Can you work these out from the model? Positions are in its coordinate system, mm. Face numbers are marked on the shaded views. A direction names the side the tool comes from. Give positions to 0.01 mm unless a question says otherwise; leave off trailing zeros. Order: outer loops, then holes, each group sorted by start corner. A loop starts at its lowest first (then second) coordinate and runs counter-clockwise, first axis right, second up. Notation, with made-up numbers: (-19, 49.5) -> (-9, 49.5) arc R31 cw to (-9, 73.5) -> close; hole circle Ø11 at (71, -1.5). An arc over 180 degrees is marked (long way). Answer as CSV lines item,"result".
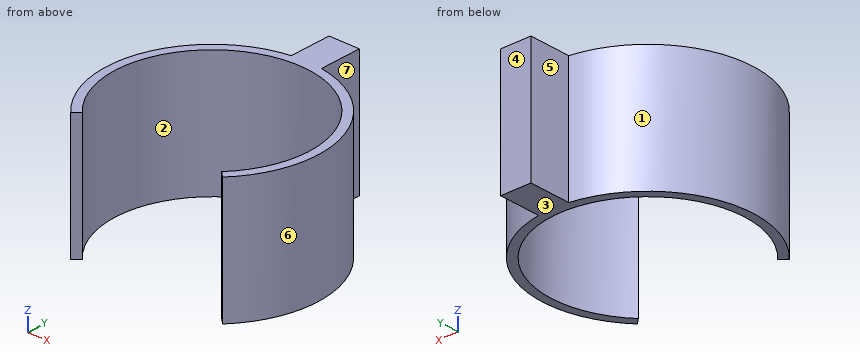
```python
from build123d import *

# Parameters (mm, degrees)
SKETCH1_R           = 4.25
SKETCH1_R_2         = 3.9
BOSS_EXTRUDE1_DEPTH = 5
CUT_EXTRUDE1_DEPTH  = 5
SKETCH3_W           = 1.224263259
SKETCH3_H           = 5
BOSS_EXTRUDE2_DEPTH = 2


with BuildPart() as part:
    # Sketch1 → Boss-Extrude1 (new body)
    with BuildSketch(Plane.XY):
        Circle(SKETCH1_R)
        Circle(SKETCH1_R_2, mode=Mode.SUBTRACT)
    extrude(amount=BOSS_EXTRUDE1_DEPTH)

    # Sketch2 → Cut-Extrude1 (cut)
    with BuildSketch(Plane.XY.offset(5)):
        with BuildLine():
            Line((-3.074069072, -2.934723044), (-2.820910442, -2.69303997))
            ThreePointArc((-2.820910442, -2.69303997), (0, -3.9), (2.820910442, -2.69303997))
            Line((2.820910442, -2.69303997), (3.074069072, -2.934723044))
            ThreePointArc((3.074069072, -2.934723044), (0, -4.25), (-3.074069072, -2.934723044))
        make_face()
    extrude(amount=-CUT_EXTRUDE1_DEPTH, mode=Mode.SUBTRACT)

    # Sketch3 → Boss-Extrude2 (add)
    with BuildSketch(Plane(origin=(0, 3.9, 0), x_dir=(1, 0, 0), z_dir=(0, 1, 0))):
        with Locations((0.012871952, -2.5)):
            Rectangle(SKETCH3_W, SKETCH3_H)
    extrude(amount=BOSS_EXTRUDE2_DEPTH)


solid = part.part
```
Item 1: Imagine slicing it at B-B, the plane z = 4.1. Please give me the cut outline in (x, y) (3 decimals).
Numbers:
outline,"(-3.074, -2.935) -> (-2.821, -2.693) arc R3.9 cw (long way) to (2.821, -2.693) -> (3.074, -2.935) arc R4.25 ccw to (0.625, 4.204) -> (0.625, 5.9) -> (-0.599, 5.9) -> (-0.599, 4.208) arc R4.25 ccw to start"
Item 2: Imagine slicing it at C-C, the plane x = 0. Please give me the cut outline in (y, z), then the cut area to 3 significant figures.
Numbers:
outline,"(3.9, 0) -> (5.9, 0) -> (5.9, 5) -> (3.9, 5) -> close"
area,"10.0 mm²"
Item 3: For pin 1 (3 mm diameter, centred on x = 2.5, z = 3, fed in from -Y); pin 2 (0.5 mm diameter, centred on y = 4.5, z = 2.5, fed in from -X); pin 3 (0.5 mm diameter, centred on y = 5, z = 3, fed in from +X) (3 decimals), each with a flat end and sliding along its axis, tell me the tip position at first contact or that it passes through.
Numbers:
pin 1,"stops at y = -2.93"
pin 2,"stops at x = -0.6"
pin 3,"stops at x = 0.625"
Item 4: For the marked faces 5, 6 and 7, which set-ups out of +Z, -Z, +X, -X, +Y, -Y let a thin tool reach every point of the face, with its end or its side?
Numbers:
face 5,"+Z, -Z, -X, +Y"
face 6,"+Z, -Z, +X"
face 7,"+Z, -Z, +X, +Y"
Item 5: Please list where these lines run through material, in increasing order: line 1 along X through (y, z) = (0, 2.4); line 2 along Y through (x, z) = (3.25, 0.7); line 3 along Y through (x, z) = (3.5, 4.7).
Numbers:
line 1,"x = -4.25 to -3.9, 3.9 to 4.25"
line 2,"y = -2.74 to -2.16, 2.16 to 2.74"
line 3,"y = -2.41 to -1.72, 1.72 to 2.41"
Item 6: Imagine slicing it at D-D, the plane y = 4.5. Please give me the cut outline in (x, z) (3 decimals), then the cut area to 3 significant figures.
Numbers:
outline,"(-0.599, 0) -> (0.625, 0) -> (0.625, 5) -> (-0.599, 5) -> close"
area,"6.12 mm²"
Item 7: Imagine slicing it at A-A, the plane y = 0. Please give me the cut outline in (x, z), then the cut area to 3 significant figures.
Numbers:
outline,"(-4.25, 0) -> (-3.9, 0) -> (-3.9, 5) -> (-4.25, 5) -> close; (3.9, 0) -> (4.25, 0) -> (4.25, 5) -> (3.9, 5) -> close"
area,"3.50 mm²"
Item 8: We'd pull the mould along Y, two halves only. Please class the marked faces 1, 2, 3 and 4: released by +Y, released by -Y, zero draft, split by the parting line, or undercut.
Numbers:
face 1,"split by the parting line"
face 2,"undercut"
face 3,"zero draft"
face 4,"released by +Y"
